from build123d import *

# Parameters (mm, degrees)
SKETCH2_R           = 17.6
BOSS_EXTRUDE1_DEPTH = 52.5
SKETCH3_R           = 2
BOSS_EXTRUDE2_DEPTH = 7.6
SKETCH4_W           = 2.5
SKETCH4_H           = 16
BOSS_EXTRUDE3_DEPTH = 3.5
CUT_EXTRUDE1_START  = -3
SKETCH5_R           = 17.6
SKETCH5_R_2         = 4.5
SKETCH5_W           = 2.5
SKETCH5_H           = 16
SKETCH5_R_3         = 2.5
CUT_EXTRUDE1_DEPTH  = 3
SKETCH7_R           = 19.95
BOSS_EXTRUDE5_DEPTH = 5.5
FILLET3_R           = 5
FILLET4_R           = 0.5


with BuildPart() as part:
    # Sketch2 → Boss-Extrude1 (new body)
    with BuildSketch(Plane.XY):
        Circle(SKETCH2_R)
    extrude(amount=BOSS_EXTRUDE1_DEPTH)

    # Sketch3 → Boss-Extrude2 (add)
    # profile 1 of 2: a face of its own
    with BuildSketch(Plane.XY):
        with BuildLine():
            Line((-14.793995556, 9.534028294), (-25.095041698, 3.292766105))
            ThreePointArc((-25.095041698, 3.292766105), (-26.95, 0), (-25.095041698, -3.292766105))
            Line((-25.095041698, -3.292766105), (-14.793995556, -9.534028294))
            ThreePointArc((-14.793995556, -9.534028294), (-17.6, 0), (-14.793995556, 9.534028294))
        make_face()
        with Locations(Location((-23.1, 0, 0), (0, 0, 180))):
            Circle(SKETCH3_R, mode=Mode.SUBTRACT)
    # profile 2 of 2: a face of its own
    with BuildSketch(Plane.XY):
        with BuildLine():
            Line((25.095041698, 3.292766105), (14.793995556, 9.534028294))
            ThreePointArc((14.793995556, 9.534028294), (17.6, 0), (14.793995556, -9.534028294))
            Line((14.793995556, -9.534028294), (25.095041698, -3.292766105))
            ThreePointArc((25.095041698, -3.292766105), (26.95, 0), (25.095041698, 3.292766105))
        make_face()
        with Locations(Location((23.1, 0, 0), (0, 0, 180))):
            Circle(SKETCH3_R, mode=Mode.SUBTRACT)
    extrude(amount=BOSS_EXTRUDE2_DEPTH)

    # Sketch4 → Boss-Extrude3 (add)
    with BuildSketch(Plane.XY.offset(52.5)):
        Rectangle(SKETCH4_W, SKETCH4_H)
    extrude(amount=BOSS_EXTRUDE3_DEPTH)

    # Sketch5 → Cut-Extrude1 (cut)
    # profile 1 of 3: a face of its own
    with BuildSketch(Plane.XY.offset(52.5).offset(CUT_EXTRUDE1_START)):
        with Locations(Location((0, 0, 0), (0, 0, 147.200140228))):
            Circle(SKETCH5_R)
        with Locations((-8.9, 0)):
            Circle(SKETCH5_R_2, mode=Mode.SUBTRACT)
        with Locations((8.9, 0)):
            Circle(SKETCH5_R_2, mode=Mode.SUBTRACT)
        Rectangle(SKETCH5_W, SKETCH5_H, mode=Mode.SUBTRACT)
    # profile 2 of 3: a face of its own
    with BuildSketch(Plane.XY.offset(52.5).offset(CUT_EXTRUDE1_START)):
        with Locations((-8.9, 0)):
            Circle(SKETCH5_R_3)
    # profile 3 of 3: a face of its own
    with BuildSketch(Plane.XY.offset(52.5).offset(CUT_EXTRUDE1_START)):
        with Locations((8.9, 0)):
            Circle(SKETCH5_R_3)
    extrude(amount=CUT_EXTRUDE1_DEPTH, mode=Mode.SUBTRACT)

    # Sketch7 → Boss-Extrude5 (add)
    with BuildSketch(Plane.XY.offset(49.5)):
        Circle(SKETCH7_R)
    extrude(amount=-BOSS_EXTRUDE5_DEPTH)

    # Fillet3
    # the kernel refuses this fillet: 5 mm, written as the material it adds along each edge
    with BuildSketch(Plane(origin=(0, 0, 44), x_dir=(1, 0, 0), z_dir=(0, 1, 0))) as fillet3_piece_1:
        with BuildLine():
            CenterArc((22.6, 4.239988208), FILLET3_R, 180, 57.994545172)
            Line((19.95, 0), (19.897, -0.084799764))
            ThreePointArc((19.897, -0.084799764), (18.775, -0.1), (17.6, -0.1))
            Line((17.6, -0.1), (17.5, 0))
            Line((17.5, 0), (17.5, 4.239988208))
            Line((17.5, 4.239988208), (17.6, 4.239988208))
        make_face()
    revolve(axis=Axis((0, 0, 44), (0, 0, -1)))

    # Fillet4
    fillet4_edges = [part.edges().sort_by_distance(p)[0] for p in [
        (1.25, 0, 56),
        (0, 8, 56),
        (0, -8, 56),
        (-1.25, 0, 56),
        (0, 8, 49.5),
        (-1.25, 0, 49.5),
        (0, -8, 49.5),
        (1.25, 0, 49.5),
        (-13.4, 0, 49.5),
        (4.4, 0, 49.5),
        (-19.95, 0, 49.5),
    ]]
    fillet(fillet4_edges, radius=FILLET4_R)


solid = part.part
Can you work these out from the model? Positions are in its coordinate system, mm. A direction names the side the tool comes from. Coordinates: 2 decimals unless noted, no trailing zeros. Write each loop counter-clockwise with the first axis right and the second up, starting at its lowest first coordinate (ties: lowest second). Pieces come first, ordered by that corner, then holes.
Q1. Imagine slicing it at B-B, the plane x = 0. List the corners of the cut face in (y, z) for me, plus the area to 3 significant figures.
Results found:
outline: (-19.95, 44) arc R5 cw to (-17.6, 39.76) - (-17.6, 0) - (17.6, 0) - (17.6, 39.76) arc R5 cw to (19.95, 44) - (19.95, 49) arc R0.5 ccw to (19.45, 49.5) - (8.5, 49.5) arc R0.5 cw to (8, 50) - (8, 55.5) arc R0.5 ccw to (7.5, 56) - (-7.5, 56) arc R0.5 ccw to (-8, 55.5) - (-8, 50) arc R0.5 cw to (-8.5, 49.5) - (-19.45, 49.5) arc R0.5 ccw to (-19.95, 49) - close
area: 1,880 mm2
Q2. For P1, Ø0.8, axis at x = -0.5, z = 52, coming from the +Y side; P2, Ø12, axis at y = 14, z = 47, coming from the +X side; P3, Ø2, axis at x = -0.5, z = 52, coming from the -Y side; P4, Ø19.5, axis at x = -9, y = -8, coming from the +Z side, each with a flat end and sliding along its axis, tell me the tip position at first contact or that it passes through.
Results found:
P1: stops at y = 8
P2: stops at x = 18.28
P3: stops at y = -8
P4: stops at z = 56
Q3. Imagine slicing it at C-C, the plane z = 29. List the corners of the cut face in (x, y) for me, plus the area to 3 significant figures.
Results found:
outline: circle Ø35.2 at (0, 0)
area: 973 mm2
Q4. If we mould it in two halves opening along Y, with no side actions, what happens to faces 6 (the face through (-1.25, 0, 53)), 7 (the face through (26.95, -0.06, 3.75)), 8 (the face through (-9, 0, 49.5))? For each: +Y half, -Y half, draft (parallel to the pull), parting line (faces both ways), or undercut.
Results found:
face 6: draft
face 7: parting line
face 8: undercut
Q5. Please list where these lines run through material, in increasing order: L1, parallel to Y at x = 23.1, z = 5.75; L2, parallel to Z at x = -1, y = 11.5; L3, parallel to Y at x = 23, z = 2.
Results found:
L1: y = -4.5 to -2, 2 to 4.5
L2: z = 0 to 49.5
L3: y = -4.56 to -2, 2 to 4.56
Q6. Which directions (+Z, -Z, +X, -X, +Y, -Y) give clear straight access to the entire face, cutting with the end or side of a thin tool? Please do faces 1 (the face through (-19.87, 6.46, 3.75)), 2 (the face through (0, 8, 53)), 3 (the face through (19.87, -6.46, 3.75)), 4 (the face through (19.03, 5.99, 46.54)), 5 (the face through (0, -8, 53)).
Results found:
face 1: -Z, -X, +Y
face 2: +Z, +X, -X, +Y
face 3: -Z, +X, -Y
face 4: +Z
face 5: +Z, +X, -X, -Y
Q7. Imagine slicing it at A-A, the plane x = 23.1. List the corners of the cut face in (y, z) for me, plus the area to 3 significant figures.
Results found:
outline: (-4.5, 0) - (-2, 0) - (-2, 7.6) - (-4.5, 7.6) - close; (2, 0) - (4.5, 0) - (4.5, 7.6) - (2, 7.6) - close
area: 38.0 mm2
